from build123d import *

# Parameters (mm, degrees)
SKETCH1_W           = 51
SKETCH1_H           = 29
BOSS_EXTRUDE1_DEPTH = 41
SKETCH2_R           = 10
SKETCH2_R_2         = 9
BOSS_EXTRUDE2_DEPTH = 1
SKETCH3_W           = 13.9
SKETCH3_H           = 12.4
CUT_EXTRUDE1_DEPTH  = 57.782479692
SKETCH4_R           = 1.5
CUT_EXTRUDE2_DEPTH  = 5


with BuildPart() as part:
    # Sketch1 → Boss-Extrude1 (new body)
    with BuildSketch(Plane(origin=(0, 0, 0), x_dir=(1, 0, 0), z_dir=(0, 1, 0))):
        Rectangle(SKETCH1_W, SKETCH1_H)
    extrude(amount=BOSS_EXTRUDE1_DEPTH)

    # Sketch2 → Boss-Extrude2 (add)
    with BuildSketch(Plane(origin=(25.5, 0, 0), x_dir=(0, 0, -1), z_dir=(1, 0, 0))):
        with Locations(Location((0, 17, 0), (0, 0, 180))):
            Circle(SKETCH2_R)
        with Locations((0, 17)):
            Circle(SKETCH2_R_2, mode=Mode.SUBTRACT)
    extrude(amount=BOSS_EXTRUDE2_DEPTH)

    # Sketch3 → Cut-Extrude1 (cut, through all)
    with BuildSketch(Plane.XY.offset(14.5)):
        with Locations((-8.95, 34.8)):
            Rectangle(SKETCH3_W, SKETCH3_H)
    extrude(amount=-CUT_EXTRUDE1_DEPTH, mode=Mode.SUBTRACT)

    # Sketch4 → Cut-Extrude2 (cut)
    with BuildSketch(Plane(origin=(0, 0, -14.5), x_dir=(-1, 0, 0), z_dir=(0, 0, -1))):
        with Locations((-18.5, 34)):
            Circle(SKETCH4_R)
        with Locations((18.5, 7)):
            Circle(SKETCH4_R)
    extrude(amount=-CUT_EXTRUDE2_DEPTH, mode=Mode.SUBTRACT)


solid = part.part
Check sheet for the modelled part. Datum: model origin and axes. Units: mm. A direction names the side the tool comes from. Round coordinates to 2 decimals unless told otherwise and drop trailing zeros. Loops run counter-clockwise (first coordinate to the right, second up) from the corner with the lowest first, then second, coordinate; pieces in that order, holes last.
1. Set-up check for faces 4 (the flat face through (-21, 41, 0)), 5 (the flat face through (-18, 7, -9.5)), 6 (the cylindrical face through (25.993, 25.923, 1.172)), 7 (the flat face through (-2, 35, 0)), 8 (the flat face through (0, 0, 0)): record each of +Z, -Z, +X, -X, +Y, -Y from which the full face is reachable in a straight line by a thin tool's end or side.
2. Sectioned sample at A-A on z = 0. Record the boundary of the cut face in (x, y).
3. Mould release check, pull along Y, two halves, no side actions. Record for faces 1 (the cylindrical face through (-17, 7, -12)), 2 (the flat face through (12, 41, 0)), 3 (the flat face through (0, 20, -14.5)): released by +Y, released by -Y, zero draft, split by the parting line, or undercut.
4. Gauge pin test, flat ends, axial feed: pin 1 Ø0.9 at (x, y) = (18.5, 34) entering from -Z; pin 2 Ø4 at (x, z) = (-10, 0.5) entering from +Y; pin 3 Ø12 at (y, z) = (16.5, 2.5) entering from +X. Record the tip position at first contact, or that the pin passes through.
5. Sectioned sample at D-D on z = -4. Record the boundary of the cut face in (x, y).
6. Sectioned sample at C-C on z = 12. Record the boundary of the cut face in (x, y), and give its area (3 significant figures).
7. Sectioned sample at B-B on y = 17. Record the boundary of the cut face in (x, z).
8. Scan lines: probe 1 along X at (y, z) = (29.5, -9); probe 2 along Y at (x, z) = (18.5, -12.65); probe 3 along Y at (x, z) = (25.8, 0). Record each from-to range of solid material in increasing order.
Recorded:
1. face 4: +Z, -Z, +X, -X, +Y
1. face 5: -Z
1. face 6: +X
1. face 7: +Z, -Z, +Y
1. face 8: +Z, -Z, +X, -X, -Y
2. outline: (-25.5, 0) - (25.5, 0) - (25.5, 7) - (26.5, 7) - (26.5, 8) - (25.5, 8) - (25.5, 26) - (26.5, 26) - (26.5, 27) - (25.5, 27) - (25.5, 41) - (-2, 41) - (-2, 28.6) - (-15.9, 28.6) - (-15.9, 41) - (-25.5, 41) - close
3. face 1: undercut
3. face 2: released by +Y
3. face 3: zero draft
4. pin 1: stops at z = -9.5
4. pin 2: stops at y = 28.6
4. pin 3: stops at x = 25.5
5. outline: (-25.5, 0) - (25.5, 0) - (25.5, 7.83) - (26.5, 7.83) - (26.5, 8.94) - (25.5, 8.94) - (25.5, 25.06) - (26.5, 25.06) - (26.5, 26.17) - (25.5, 26.17) - (25.5, 41) - (-2, 41) - (-2, 28.6) - (-15.9, 28.6) - (-15.9, 41) - (-25.5, 41) - close
6. outline: (-25.5, 0) - (25.5, 0) - (25.5, 41) - (-2, 41) - (-2, 28.6) - (-15.9, 28.6) - (-15.9, 41) - (-25.5, 41) - close
6. area: 1,920 mm2
7. outline: (-25.5, -14.5) - (25.5, -14.5) - (25.5, -10) - (26.5, -10) - (26.5, -9) - (25.5, -9) - (25.5, 9) - (26.5, 9) - (26.5, 10) - (25.5, 10) - (25.5, 14.5) - (-25.5, 14.5) - close
8. probe 1: x = -25.5 to -15.9, -2 to 25.5
8. probe 2: y = 0 to 32.5, 35.5 to 41
8. probe 3: y = 7 to 8, 26 to 27
